Design review of the part built by this model. Coordinates are the model's own, in mm. Face numbers are marked on the shaded views. A direction names the side the tool comes from. Give positions to 0.01 mm unless a question says otherwise; leave off trailing zeros. Loops run counter-clockwise (first coordinate to the right, second up) from the corner with the lowest first, then second, coordinate; pieces in that order, holes last. Notation, with made-up numbers: (31.5, 64) - (73.5, 64) arc R16 ccw to (73.5, 91) - close; hole circle Ø8 at (73, 2). An arc over 180 degrees is marked (long way). One line per item, written item: value. Start each with the question number.
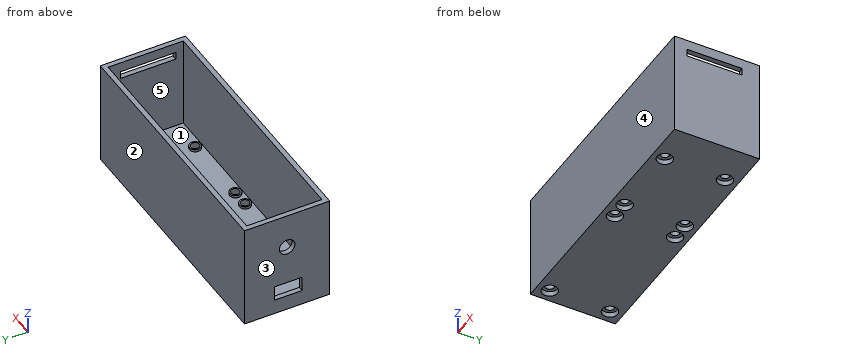
```python
from build123d import *

# Parameters (mm, degrees)
SKETCH_W          = 100
SKETCH_H          = 30
PAD_DEPTH         = 40
THICKNESS_T       = 2
THICKNESS_FACE5_W = 30
THICKNESS_FACE5_H = 100
PAD001_DEPTH      = 3
SKETCH001_R       = 2.25
PAD002_DEPTH      = 1
HOLE_D            = 3.4
HOLE_DEPTH        = 25
HOLE_CBORE_D      = 6.1
HOLE_CBORE_DEPTH  = 2
SKETCH003_W       = 22
SKETCH003_H       = 3
POCKET_DEPTH      = 2
SKETCH004_R       = 3.1
SKETCH004_W       = 11
SKETCH004_H       = 6
POCKET001_DEPTH   = 2


with BuildPart() as part:
    # Sketch → Pad (new body)
    with BuildSketch(Plane.XY):
        Rectangle(SKETCH_W, SKETCH_H)
    extrude(amount=PAD_DEPTH)

    # Thickness
    thickness_openings = [part.faces().sort_by_distance(p)[0] for p in [
        (0, 0, 40),
    ]]
    offset(amount=THICKNESS_T, openings=thickness_openings, kind=Kind.INTERSECTION)

    # Thickness Face5 → Pad001 (add)
    with BuildSketch(Plane(origin=(0, 0, 0), x_dir=(0, 1, 0), z_dir=(0, 0, 1))):
        Rectangle(THICKNESS_FACE5_W, THICKNESS_FACE5_H)
    extrude(amount=PAD001_DEPTH)

    # Sketch001 (on Face2 of Pad001) → Pad002 (join)
    with BuildSketch(Plane.XY.offset(3)):
        with Locations((-47, 12)):
            Circle(SKETCH001_R)
        with Locations((0, 12)):
            Circle(SKETCH001_R)
        with Locations((7, 12)):
            Circle(SKETCH001_R)
        with Locations((36, 12)):
            Circle(SKETCH001_R)
        with Locations((-47, -12)):
            Circle(SKETCH001_R)
        with Locations((0, -12)):
            Circle(SKETCH001_R)
        with Locations((7, -12)):
            Circle(SKETCH001_R)
        with Locations((36, -12)):
            Circle(SKETCH001_R)
    extrude(amount=PAD002_DEPTH)

    # Hole
    with Locations(Plane(origin=(0, 0, -2), x_dir=(1, 0, 0), z_dir=(0, 0, -1))):
        with Locations((-47, 12), (0, 12), (7, 12), (36, 12), (-47, -12), (0, -12), (7, -12), (36, -12)):
            CounterBoreHole(HOLE_D / 2, HOLE_CBORE_D / 2, HOLE_CBORE_DEPTH, depth=HOLE_DEPTH)

    # Sketch003 (on Face18 of Hole) → Pocket (cut)
    with BuildSketch(Plane.YZ.offset(52)):
        with Locations((-1, 34.5)):
            Rectangle(SKETCH003_W, SKETCH003_H)
    extrude(amount=-POCKET_DEPTH, mode=Mode.SUBTRACT)

    # Sketch004 (on Face20 of Pocket) → Pocket001 (cut)
    with BuildSketch(Plane(origin=(-52, 0, 0), x_dir=(0, -1, 0), z_dir=(-1, 0, 0))):
        with Locations((0, 26)):
            Circle(SKETCH004_R)
        with Locations((0.5, 7)):
            Rectangle(SKETCH004_W, SKETCH004_H)
    extrude(amount=-POCKET001_DEPTH, mode=Mode.SUBTRACT)


solid = part.part
```
(1) Draft analysis for pull direction X (two halves, no side actions). For the marked faces 1, 2 and 3, state which applies: pulls with the +X half, pulls with the -X half, needs draft (parallel to the pull), parting line crosses it, or undercut.
(2) Take a section at C-C on x = 7. State how many separate pieces and enclosed holes the cut face has, and give its area (3 significant figures).
(3) Take a section at D-D on z = 37. State the section outline as (x, y) points.
(4) For pin 1 Ø8 at (x, y) = (-47, 12) entering from -Z; pin 2 Ø4 at (x, y) = (35, -9.5) entering from +Z; pin 3 Ø5 at (x, y) = (0, -12) entering from -Z, all flat-tipped, find the tip position at first contact; note any pin that passes through.
(5) Machinability: for the marked faces 4 and 5, which of the approach directions +Z, -Z, +X, -X, +Y, -Y give a long, thin tool a straight path to every point of the face, cutting with its end or side? Answer none if there is none.
(6) Take a section at A-A on y = 8. State the section outline as (x, z) points.
(7) To check wall thickness, follow L1, parallel to X at y = -12, z = 0.95; L2, parallel to X at y = -12, z = -0.85; L3, parallel to Y at x = 7, z = -1. State the ranges of each line that lie inside material, in increasing order. Write a range as from..to.
(8) Take a section at B-B on y = 0. State the section outline as (x, z) points.
Here are the results:
1. face 1: undercut
1. face 2: needs draft
1. face 3: pulls with the -X half
2. separate pieces: 3
2. enclosed holes: 0
2. area: 275 mm²
3. outline: (-52, -17) - (52, -17) - (52, 17) - (-52, 17) - close; hole (-50, -15) - (50, -15) - (50, 15) - (-50, 15) - close
4. pin 1: z = -2
4. pin 2: z = 4
4. pin 3: z = 0
5. face 4: +Z, -Z, +X, -X, -Y
5. face 5: +Z
6. outline: (-52, -2) - (52, -2) - (52, 33) - (50, 33) - (50, 3) - (-50, 3) - (-50, 40) - (-52, 40) - close; (50, 36) - (52, 36) - (52, 40) - (50, 40) - close
7. L1: -52..-48.7, -45.3..-1.7, 1.7..5.3, 8.7..34.3, 37.7..52
7. L2: -52..-50.05, -43.95..-3.05, 3.05..3.95, 10.05..32.95, 39.05..52
7. L3: -17..-15.05, -8.95..8.95, 15.05..17
8. outline: (-52, -2) - (52, -2) - (52, 33) - (50, 33) - (50, 3) - (-50, 3) - (-50, 4) - (-52, 4) - close; (-52, 10) - (-50, 10) - (-50, 22.9) - (-52, 22.9) - close; (-52, 29.1) - (-50, 29.1) - (-50, 40) - (-52, 40) - close; (50, 36) - (52, 36) - (52, 40) - (50, 40) - close
